The model under review builds one solid part; all positions refer to its coordinate system, in mm. A direction names the side the tool comes from. Coordinates: 2 decimals unless noted, no trailing zeros. Order: outer loops, then holes, each group sorted by start corner. A loop starts at its lowest first (then second) coordinate and runs counter-clockwise, first axis right, second up. Notation, with made-up numbers: (3, -6) -> (35, -6) arc R24 ccw to (35, 9) -> close; hole circle Ø1 at (72.5, 75.25). An arc over 180 degrees is marked (long way). Use one line per item in the form item = value.
from build123d import *

# Parameters (mm, degrees)
F0_W     = 76.2
F0_H     = 50.8
F1_DEPTH = 50.8
F3_DEPTH = 81.788
F4_W     = 44.9072
F4_H     = 51.87745
F5_DEPTH = 47.244


with BuildPart() as f1:
    # F0 (on Top) → F1 (new body)
    with BuildSketch(Plane.XY):
        with Locations((0.774292, -7.57095)):
            Rectangle(F0_W, F0_H)
    extrude(amount=F1_DEPTH)

    # F2 (on face) → F3 (cut)
    with BuildSketch(Plane(origin=(-37.325708, 0, 0), x_dir=(0, -1, 0), z_dir=(-1, 0, 0))):
        Polygon((-17.82905, 23.158375), (8.392135, 50.8), (-17.82905, 50.8), align=None)
    extrude(amount=-F3_DEPTH, mode=Mode.SUBTRACT)

    # F4 (on Front) → F5 (cut)
    with BuildSketch(Plane.XZ):
        with Locations((1.031568, 25.938725)):
            Rectangle(F4_W, F4_H)
    extrude(amount=-F5_DEPTH, mode=Mode.SUBTRACT)


solid = f1.part
Item 1: We need section D-D (z = 35). Write out the cut boundary in (x, y), plus the area to 3 significant figures.
Results found:
outline = (-37.33, -32.97) -> (38.87, -32.97) -> (38.87, 6.6) -> (23.49, 6.6) -> (23.49, 0) -> (-21.42, 0) -> (-21.42, 6.6) -> (-37.33, 6.6) -> close
area = 2,720 mm²
Item 2: We need section A-A (y = 8.5). Write out the cut boundary in (x, z), plus the area to 3 significant figures.
Results found:
outline = (-37.33, 0) -> (-21.42, 0) -> (-21.42, 32.99) -> (-37.33, 32.99) -> close; (23.49, 0) -> (38.87, 0) -> (38.87, 32.99) -> (23.49, 32.99) -> close
area = 1,030 mm²
Item 3: We need section B-B (z = 21). Write out the cut boundary in (x, y), plus the area to 3 significant figures.
Results found:
outline = (-37.33, -32.97) -> (38.87, -32.97) -> (38.87, 17.83) -> (23.49, 17.83) -> (23.49, 0) -> (-21.42, 0) -> (-21.42, 17.83) -> (-37.33, 17.83) -> close
area = 3,070 mm²
Item 4: Draft analysis for pull direction X (two halves, no side actions). For faces 3 (the face through (1, 0, 21)), 4 (the face through (-21.422, 9, 16)), 5 (the face through (0.2, -0.9, 42.9)), 6 (the face through (-37.326, -8, 25)), state which applies: released by +X, released by -X, zero draft, split by the parting line, or undercut.
Results found:
face_3 = undercut
face_4 = undercut
face_5 = zero draft
face_6 = released by -X
Item 5: We need section C-C (x = -1). Write out the cut boundary in (y, z), plus the area to 3 significant figures.
Results found:
outline = (-32.97, 0) -> (0, 0) -> (0, 41.95) -> (-8.39, 50.8) -> (-32.97, 50.8) -> close
area = 1,640 mm²
Item 6: To check wall thickness, follow L1, parallel to X at y = 4, z = 26.5; L2, parallel to Y at x = -1, z = 29; L3, parallel to Z at x = -24, y = 0. State the ranges of each line that lie inside material, in increasing order. Write a range as from..to.
Results found:
L1 = -37.33..-21.42, 23.49..38.87
L2 = -32.97..0
L3 = 0..41.95
Item 7: Clearance check with a flat-ended pin moving along its axis: pin 1 (21 mm diameter, centred on x = -7.5, z = 22, fed in from +Y). State where the tip first meets the part, or that it passes through.
Results found:
pin_1 = 0
Item 8: Tool access review of faces 1 (the face through (31, 17.829, 11)), 2 (the face through (23.485, 9, 16)): name each direction out of +Z, -Z, +X, -X, +Y, -Y from which nothing blocks a thin tool from reaching the whole face with its end or side.
Results found:
face_1 = +Z, -Z, +X, -X, +Y
face_2 = +Z, -Z, +Y
